```python
from build123d import *

# Parameters (mm, degrees)
F0_W      = 175.26
F0_H      = 50.8
F0_W_2    = 28.829
F0_H_2    = 13.5255
F0_W_3    = 28.7655
F1_DEPTH  = 46.99
F2_R      = 12.954
F3_DEPTH  = 76.2
F4_DEPTH  = 25.4
F5_R      = 12.573
F5_R_2    = 9.779
F6_DEPTH  = 76.2
F7_DEPTH  = 25.4
F8_R      = 11.43
F9_DEPTH  = 76.2
F10_DEPTH = 25.4
F11_R     = 13.1445
F11_R_2   = 10.3505
F12_DEPTH = 76.2
F13_DEPTH = 25.4


with BuildPart() as f1:
    # F0 (on Front) → F1 (new body)
    with BuildSketch(Plane.XZ):
        Rectangle(F0_W, F0_H)
        with Locations((-61.2013, 0)):
            Rectangle(F0_W_2, F0_H_2, mode=Mode.SUBTRACT)
        with Locations((-20.3581, 0)):
            Rectangle(F0_W_2, F0_H_2, mode=Mode.SUBTRACT)
        with Locations((20.45335, 0)):
            Rectangle(F0_W_3, F0_H_2, mode=Mode.SUBTRACT)
        with Locations((61.23305, 0)):
            Rectangle(F0_W_3, F0_H_2, mode=Mode.SUBTRACT)
    extrude(amount=F1_DEPTH)

    # F2 (on face) → F3 (join)
    with BuildSketch(Plane.XY.offset(25.4)):
        with BuildLine():
            ThreePointArc((60.96, 0), (49.8244824099, -26.8835175901), (76.708, -15.748))
            ThreePointArc((76.708, -15.748), (72.0955175901, -4.6124824099), (60.96, 0))
        make_face()
        with Locations((60.96, -15.748)):
            Circle(F2_R, mode=Mode.SUBTRACT)
    extrude(amount=F3_DEPTH)

    # F4 (cut): a face of the model
    f4_faces = [f1.faces().sort_by_distance(p)[0] for p in [
        (60.96, -15.748, 25.4),
    ]]
    extrude(f4_faces, amount=-F4_DEPTH, mode=Mode.SUBTRACT)

    # F5 (on face) → F6 (join)
    with BuildSketch(Plane.XY.offset(25.4)):
        with Locations((20.32, -12.573)):
            Circle(F5_R)
        with Locations((20.32, -12.573)):
            Circle(F5_R_2, mode=Mode.SUBTRACT)
    extrude(amount=F6_DEPTH)

    # F7 (cut): a face of the model
    f7_faces = [f1.faces().sort_by_distance(p)[0] for p in [
        (20.32, -12.573, 25.4),
    ]]
    extrude(f7_faces, amount=-F7_DEPTH, mode=Mode.SUBTRACT)

    # F8 (on face) → F9 (join)
    with BuildSketch(Plane.XY.offset(25.4)):
        with BuildLine():
            ThreePointArc((-20.319999941, 0), (-30.3778868765, -24.2818868347), (-6.096, -14.224))
            ThreePointArc((-6.096, -14.224), (-10.2621131235, -4.1661131653), (-20.319999941, 0))
        make_face()
        with Locations((-20.32, -14.224)):
            Circle(F8_R, mode=Mode.SUBTRACT)
    extrude(amount=F9_DEPTH)

    # F10 (cut): a face of the model
    f10_faces = [f1.faces().sort_by_distance(p)[0] for p in [
        (-20.32, -14.224, 25.4),
    ]]
    extrude(f10_faces, amount=-F10_DEPTH, mode=Mode.SUBTRACT)

    # F11 (on face) → F12 (join)
    with BuildSketch(Plane.XY.offset(25.4)):
        with Locations((-60.96, -13.1445)):
            Circle(F11_R)
        with Locations((-60.96, -13.1445)):
            Circle(F11_R_2, mode=Mode.SUBTRACT)
    extrude(amount=F12_DEPTH)

    # F13 (cut): a face of the model
    f13_faces = [f1.faces().sort_by_distance(p)[0] for p in [
        (-60.96, -13.1445, 25.4),
    ]]
    extrude(f13_faces, amount=-F13_DEPTH, mode=Mode.SUBTRACT)


solid = f1.part
```
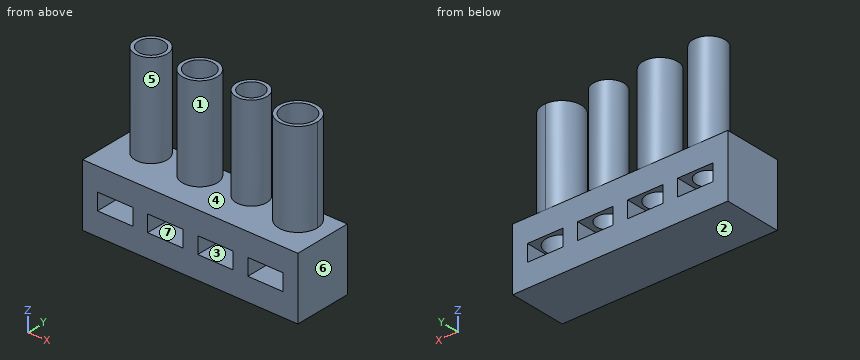
Can you work these out from the model? Positions are in its coordinate system, mm. Face numbers are marked on the shaded views. A direction names the side the tool comes from. Round coordinates to 2 decimals unless told otherwise and drop trailing zeros. Loops run counter-clockwise (first coordinate to the right, second up) from the corner with the lowest first, then second, coordinate; pieces in that order, holes last.
Item 1: Suppose I cut it at C-C, the plane x = 57. Write out the boundary of the cut face in (y, z).
Item 2: Suppose I cut it at A-A, the plane z = 85. Write out the boundary of the cut face in (x, y).
Item 3: Will these pins go through, and if not, where does the flat tip stop? pin 1 Ø3 at (x, z) = (-10.5, 65.5) entering from +Y; pin 2 Ø15.5 at (x, y) = (20.32, -12.573) entering from +Z; pin 3 Ø4 at (y, z) = (-18, 37.5) entering from -X.
Item 4: Suppose I cut it at B-B, the plane y = -37. Write out the boundary of the cut face in (x, z), then the cut area to 3 significant figures.
Item 5: Which directions (+Z, -Z, +X, -X, +Y, -Y) give clear straight access to the entire face, cutting with the end or side of a thin tool? Please do the marked faces 5, 6 and 7.
Item 6: If we mould it in two halves opening along Z, with no side actions, what happens to the marked faces 1, 2, 3 and 4? For each: +Z half, -Z half, draft (parallel to the pull), parting line (faces both ways), or undercut.
Item 7: Please list where these lines run through material, in increasing order: L1, parallel to Z at x = 31, y = -23.5; L2, parallel to Y at x = 60, z = 19; L3, parallel to Y at x = -20.32, z = 20.
Reported:
1. outline: (-46.99, -25.4) - (0, -25.4) - (0, -6.76) - (-46.99, -6.76) - close; (-46.99, 6.76) - (-28.08, 6.76) - (-28.08, 101.6) - (-30.99, 101.6) - (-30.99, 25.4) - (-46.99, 25.4) - close; (-3.41, 6.76) - (0, 6.76) - (0, 25.4) - (-0.51, 25.4) - (-0.51, 101.6) - (-3.41, 101.6) - close
2. outline: circle Ø26.29 at (-60.96, -13.14); circle Ø28.45 at (-20.32, -14.22); circle Ø25.15 at (20.32, -12.57); circle Ø31.5 at (60.96, -15.75); hole circle Ø20.7 at (-60.96, -13.14); hole circle Ø22.86 at (-20.32, -14.22); hole circle Ø19.56 at (20.32, -12.57); hole circle Ø25.91 at (60.96, -15.75)
3. pin 1: stops at y = -2.69
3. pin 2: stops at z = -6.76
3. pin 3: stops at x = -73.79
4. outline: (-87.63, -25.4) - (87.63, -25.4) - (87.63, 25.4) - (-87.63, 25.4) - close; hole (-75.62, -6.76) - (-46.79, -6.76) - (-46.79, 6.76) - (-75.62, 6.76) - close; hole (-34.77, -6.76) - (-5.94, -6.76) - (-5.94, 6.76) - (-34.77, 6.76) - close; hole (6.07, -6.76) - (34.84, -6.76) - (34.84, 6.76) - (6.07, 6.76) - close; hole (46.85, -6.76) - (75.62, -6.76) - (75.62, 6.76) - (46.85, 6.76) - close
4. area: 7,350 mm2
5. face 5: +Z
5. face 6: +Z, -Z, +X, +Y, -Y
5. face 7: +Y, -Y
6. face 1: draft
6. face 2: -Z half
6. face 3: undercut
6. face 4: +Z half
7. L1: z = -25.4 to -6.76, 6.76 to 25.4
7. L2: y = -46.99 to -28.67, -2.83 to 0
7. L3: y = -46.99 to -25.65, -2.79 to 0
